Model file for the job. Use its own axes, mm. Coordinates: 2 decimals unless noted, no trailing zeros. Write each loop counter-clockwise with the first axis right and the second up, starting at its lowest first coordinate (ties: lowest second). Pieces come first, ordered by that corner, then holes. Notation, with made-up numbers: M 1,55.25 L 35,55.25 A14 ccw 35,66.25 Z; hole C -23.5,86 d4. An arc over 180 degrees is marked long. Put each result on its own line as item: value. Start each with the question number.
Q1. Drop a flat-ended pin along its axis: pin 1 (4 mm diameter, centred on y = -2.5, z = 32, fed in from -X). Give the stop position or say it passes through.
Q2. Cut at C-C (z = 32). Write the cut outline in (x, y).
Q3. Cut at B-B (x = 21). Write the cut outline in (y, z).
Q4. Cut at A-A (y = -26). Write the cut outline in (x, z).
Q5. Drill centre lines: line 1 along Z through (x, y) = (-19, 16.5); line 2 along Z through (x, y) = (-34, 34.5); line 3 along X through (y, z) = (-29, 38.5). Where is each one in solid material? Low to high.
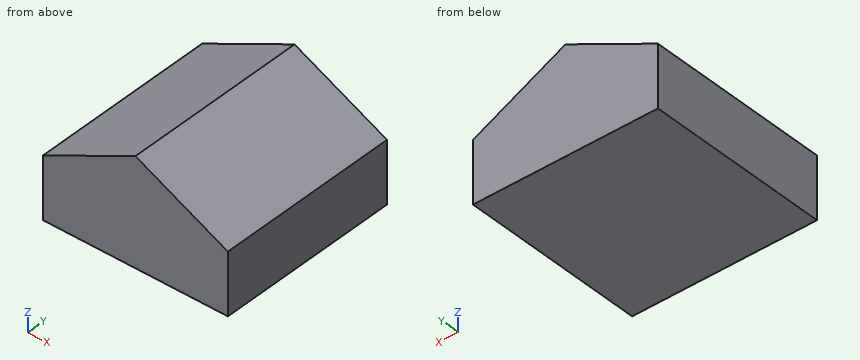
```python
from build123d import *

# Parameters (mm, degrees)
F0_W     = 76.2
F0_H     = 37.6850995183
F0_H_2   = 38.5149004817
F1_DEPTH = 25.4
F3_DEPTH = 76.2


with BuildPart() as f1:
    # F0 (on Top) → F1 (new body)
    with BuildSketch(Plane.XY):
        with Locations((-5.4470213876, 18.8425497591)):
            Rectangle(F0_W, F0_H)
        with Locations((-5.4470213876, -19.2574502409)):
            Rectangle(F0_W, F0_H_2)
    extrude(amount=F1_DEPTH)

    # F2 (on face) → F3 (join)
    with BuildSketch(Plane.XZ.offset(38.5149004817)):
        Polygon((-43.5470213876, 25.4), (32.6529786124, 25.4), (-5.4470213876, 43.9809113741), align=None)
    extrude(amount=-F3_DEPTH)


solid = f1.part
```
Computed values:
1. pin 1: x = -34.11
2. outline: M -30.01,-38.51 L 19.12,-38.51 L 19.12,37.69 L -30.01,37.69 Z
3. outline: M -38.51,0 L 37.69,0 L 37.69,31.08 L -38.51,31.08 Z
4. outline: M -43.55,0 L 32.65,0 L 32.65,25.4 L -5.45,43.98 L -43.55,25.4 Z
5. line 1: 0 to 37.37
5. line 2: 0 to 30.06
5. line 3: -16.69 to 5.79
